Study the drawing (mm; zero at the part's minimum x, y, z) and answer. A direction names the side the tool comes from. Give positions to 0.01 mm unless a question says otherwise; leave off trailing zeros. Loops run counter-clockwise (first coordinate to the right, second up) from the corner with the lowest first, then second, coordinate; pieces in that order, holes last. Notation, with made-up numbers: (41.25, -28) - (93.25, -28) arc R13 cw to (93.25, -3) - close; hole circle Ø7 at (-3.75, 76). An arc over 180 degrees is marked (long way). Answer in a Markdown table with one row per item. Add a question column.
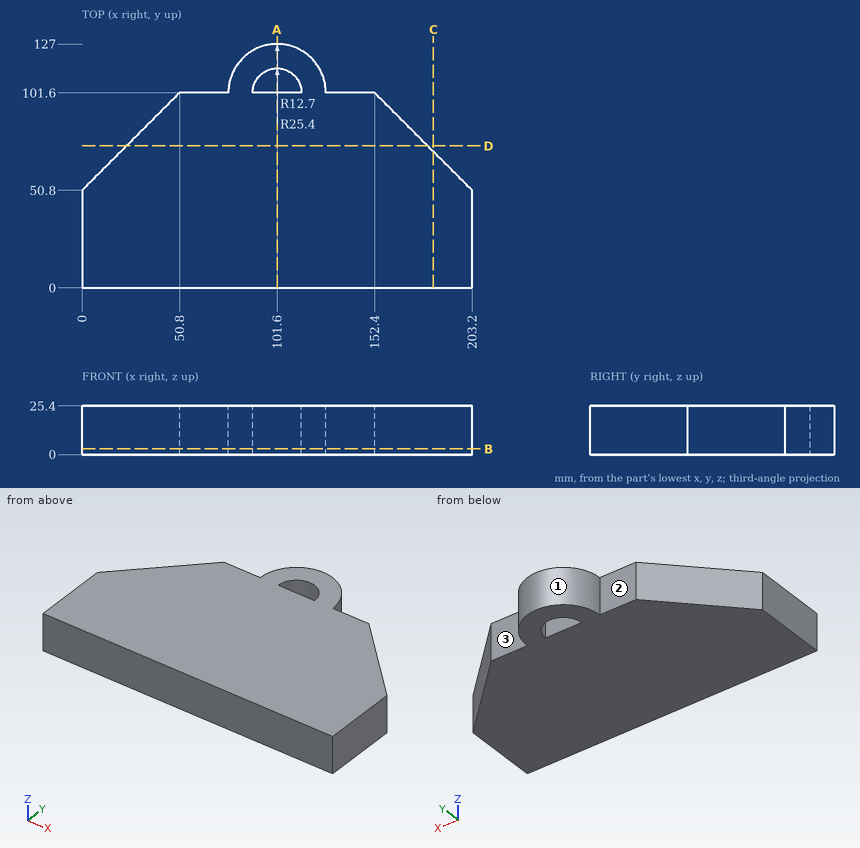
(1) A cutting plane is placed at B-B on z = 3. Determine the outline of the cut face in (x, y).
(2) Given pin 1 Ø8 at (y, z) = (56.5, 20) entering from +X; pin 2 Ø2 at (x, y) = (63.5, 32.5) entering from -Z; pin 3 Ø4 at (x, z) = (125, 6) entering from +Y; pin 4 Ø4 at (x, z) = (174, 10.5) entering from +Y, each flat-ended and moving along its own axis, determine where each tip first touches the part or whether it passes through.
(3) Find the intervals of material crossed by line 1 along Y through (x, z) = (66, 14.5); line 2 along Y through (x, z) = (14, 20.25); line 3 along X through (y, z) = (68.5, 6), in increasing order. Write a range as [from, to].
(4) A cutting plane is placed at C-C on x = 183. Determine the outline of the cut face in (y, z), plus the area to 3 significant figures.
(5) A cutting plane is placed at D-D on y = 74. Determine the outline of the cut face in (x, z), plus the area to 3 significant figures.
(6) A cutting plane is placed at A-A on x = 101.6. Determine the outline of the cut face in (y, z).
(7) A tool of negligible diameter and unlimited length cuts with its end or side. For the marked faces 1, 2 and 3, from which of +Z, -Z, +X, -X, +Y, -Y can it reach the whole face along a straight path? Write none if from no direction.
Evaluation:
| question | item | result |
|---|---|---|
| 1 | outline | (0, 0) - (203.2, 0) - (203.2, 50.8) - (152.4, 101.6) - (127, 101.6) arc R25.4 ccw to (76.2, 101.6) - (50.8, 101.6) - (0, 50.8) - close; hole (88.9, 101.6) - (114.3, 101.6) arc R12.7 ccw to start |
| 2 | pin 1 | stops at x = 201.5 |
| 2 | pin 2 | stops at z = 0 |
| 2 | pin 3 | stops at y = 115.28 |
| 2 | pin 4 | stops at y = 82 |
| 3 | line 1 | y = [0, 101.6] |
| 3 | line 2 | y = [0, 64.8] |
| 3 | line 3 | x = [17.7, 185.5] |
| 4 | outline | (0, 0) - (71, 0) - (71, 25.4) - (0, 25.4) - close |
| 4 | area | 1,800 mm² |
| 5 | outline | (23.2, 0) - (180, 0) - (180, 25.4) - (23.2, 25.4) - close |
| 5 | area | 3,980 mm² |
| 6 | outline | (0, 0) - (101.6, 0) - (101.6, 25.4) - (0, 25.4) - close; (114.3, 0) - (127, 0) - (127, 25.4) - (114.3, 25.4) - close |
| 7 | face 1 | +Z, -Z, +Y |
| 7 | face 2 | +Z, -Z, -X, +Y |
| 7 | face 3 | +Z, -Z, +X, +Y |
